from build123d import *

# Parameters (mm, degrees)
SKETCH1_W           = 40
SKETCH1_H           = 40
BOSS_EXTRUDE2_DEPTH = 9.54
SKETCH2_W           = 32
SKETCH2_H           = 32
CUT_EXTRUDE1_DEPTH  = 8
BOSS_EXTRUDE3_DEPTH = 42
CIRPATTERN1_COUNT   = 2
CIRPATTERN1_ANGLE   = 90
BOSS_EXTRUDE4_DEPTH = 34.13
CIRPATTERN2_COUNT   = 2
CIRPATTERN2_ANGLE   = 90
FILLET1_R           = 2.5
FILLET2_R           = 5


with BuildPart() as part:
    # Sketch1 → Boss-Extrude2 (new body)
    with BuildSketch(Plane(origin=(0, 0, 0), x_dir=(1, 0, 0), z_dir=(0, 1, 0))):
        Rectangle(SKETCH1_W, SKETCH1_H)
    extrude(amount=BOSS_EXTRUDE2_DEPTH)

    # Sketch2 → Cut-Extrude1 (cut)
    with BuildSketch(Plane(origin=(0, 9.54, 0), x_dir=(1, 0, 0), z_dir=(0, 1, 0))):
        Rectangle(SKETCH2_W, SKETCH2_H)
    extrude(amount=-CUT_EXTRUDE1_DEPTH, mode=Mode.SUBTRACT)

    # Sketch3 → Boss-Extrude3 (add)
    with BuildSketch(Plane(origin=(0, 1.54, 0), x_dir=(1, 0, 0), z_dir=(0, 1, 0))):
        Polygon((3.5, 20), (-3.5, 20), (-3.5, 16), (-9.25, 16), (-9.25, 14.4844), (-6.2656, 11.5), (6.2656, 11.5), (9.25, 14.4844), (9.25, 16), (3.5, 16), align=None)
    boss_extrude3 = extrude(amount=BOSS_EXTRUDE3_DEPTH)

    # CirPattern1: Boss-Extrude3 ×2 about axis
    cirpattern1_axis = Axis((0, 0, 0), (0, 1, 0))
    for i in range(1, CIRPATTERN1_COUNT):
        add(boss_extrude3.rotate(cirpattern1_axis, i * CIRPATTERN1_ANGLE / (CIRPATTERN1_COUNT - 1)))

    # Sketch4 → Boss-Extrude4 (add)
    with BuildSketch(Plane.XY.offset(20)):
        Polygon((-4.075, 0), (4.075, 0), (4.075, 4.54), (9.45, 4.54), (9.45, 7.3), (6.689745603, 9.54), (-6.689745603, 9.54), (-9.45, 7.3), (-9.45, 4.54), (-4.075, 4.54), align=None)
    boss_extrude4 = extrude(amount=BOSS_EXTRUDE4_DEPTH)

    # CirPattern2: Boss-Extrude4 ×2 about axis
    cirpattern2_axis = Axis((0, 0, 0), (0, 1, 0))
    for i in range(1, CIRPATTERN2_COUNT):
        add(boss_extrude4.rotate(cirpattern2_axis, i * CIRPATTERN2_ANGLE / (CIRPATTERN2_COUNT - 1)))

    # Fillet1
    fillet1_edges = [part.edges().sort_by_distance(p)[0] for p in [
        (16, 5.54, -16),
        (16, 5.54, 16),
        (-16, 5.54, 16),
        (-16, 5.54, -16),
    ]]
    fillet(fillet1_edges, radius=FILLET1_R)

    # Fillet2
    fillet2_edges = [part.edges().sort_by_distance(p)[0] for p in [
        (20, 4.77, 20),
        (-20, 4.77, 20),
        (-20, 4.77, -20),
        (20, 4.77, -20),
    ]]
    fillet(fillet2_edges, radius=FILLET2_R)


solid = part.part
The listing builds one solid part. Answer for the finished solid, in the listing's coordinates (mm). A direction names the side the tool comes from. Round coordinates to 2 decimals unless told otherwise and drop trailing zeros. Order: outer loops, then holes, each group sorted by start corner. A loop starts at its lowest first (then second) coordinate and runs counter-clockwise, first axis right, second up. Notation, with made-up numbers: (82.5, 38.25) - (111.5, 38.25) arc R15 cw to (111.5, 57.25) - close; hole circle Ø5 at (87.25, 58.25). An arc over 180 degrees is marked (long way). Write item = value, one per line. Start each with the question number.
1) Section A-A, the plane y = 32 is taken. Write down the section's boundary in (x, z).
2) For faces 5 (the flat face through (-16, 26, 6)), 6 (the flat face through (6, 26, -16)), 7 (the flat face through (7.737, 22.246, -12.971)), 8 (the flat face through (37, 2, -4.075)), determine the directions among +Z, -Z, +X, -X, +Y, -Y from which every point of the face is accessible in a straight line to the end or side of a thin tool.
3) For a pull along Z with two mould halves and no side action, classify faces 1 (the flat face through (37, 6, 9.45)), 2 (the flat face through (4.075, 2, 37)), 3 (the flat face through (0, 1.54, 0)), 4 (the flat face through (0, 12, -20)) as released by +Z, released by -Z, zero draft, split by the parting line, or undercut.
4) Section D-D, the plane x = -12.5 is taken. Write down the section's boundary in (y, z), plus the area to 3 significant figures.
5) Given pin 1 (5 mm diameter, centred on x = 31, y = 2.5, fed in from +Z); pin 2 (1.5 mm diameter, centred on y = 37, z = 2.5, fed in from +X); pin 3 (4.5 mm diameter, centred on x = -18.5, y = 19.5, fed in from +Z), each flat-ended and moving along its own axis, determine where each tip first touches the part or whether it passes through.
6) Section C-C, the plane z = 48 is taken. Write down the section's boundary in (x, y) (3 decimals), plus the area to 3 significant figures.
7) Section B-B, the plane x = 36.5 is taken. Write down the section's boundary in (y, z) (3 decimals), plus the area to 3 significant figures.
8) Straight lines are drawn through the part: L1, parallel to X at y = 7.5, z = -1.5; L2, parallel to X at y = 31.5, z = -1. For each, find the intervals that lie inside material, in ascending order.
Results list:
q1.outline = (-20, -3.5) - (-16, -3.5) - (-16, -9.25) - (-14.48, -9.25) - (-11.5, -6.27) - (-11.5, 6.27) - (-14.48, 9.25) - (-16, 9.25) - (-16, 3.5) - (-20, 3.5) - close; (-9.25, -16) - (-3.5, -16) - (-3.5, -20) - (3.5, -20) - (3.5, -16) - (9.25, -16) - (9.25, -14.48) - (6.27, -11.5) - (-6.27, -11.5) - (-9.25, -14.48) - close
q2.face_5 = +Z, -X, +Y
q2.face_6 = -Z, +X, +Y
q2.face_7 = +Y
q2.face_8 = -Z, +X, -Y
q3.face_1 = released by +Z
q3.face_2 = zero draft
q3.face_3 = undercut
q3.face_4 = released by -Z
q4.outline = (0, -20) - (9.54, -20) - (9.54, -16) - (1.54, -16) - (1.54, -7.27) - (43.54, -7.27) - (43.54, 7.27) - (1.54, 7.27) - (1.54, 16) - (9.54, 16) - (9.54, 20) - (0, 20) - close
q4.area = 736 mm^2
q5.pin_1 = 9.45
q5.pin_2 = -11.5
q5.pin_3 = 3.5
q6.outline = (-9.45, 4.54) - (-4.075, 4.54) - (-4.075, 0) - (4.075, 0) - (4.075, 4.54) - (9.45, 4.54) - (9.45, 7.3) - (6.69, 9.54) - (-6.69, 9.54) - (-9.45, 7.3) - close
q6.area = 125 mm^2
q7.outline = (0, -4.075) - (4.54, -4.075) - (4.54, -9.45) - (7.3, -9.45) - (9.54, -6.69) - (9.54, 6.69) - (7.3, 9.45) - (4.54, 9.45) - (4.54, 4.075) - (0, 4.075) - close
q7.area = 125 mm^2
q8.L1 = -20 to -11.5, 16 to 54.13
q8.L2 = -20 to -11.5
